```python
from build123d import *

# Parameters (mm, degrees)
F0_R     = 150
F1_DEPTH = 10
F2_R     = 150
F2_R_2   = 130
F2_R_3   = 100
F3_DEPTH = 3


with BuildPart() as f1:
    # F0 (on Top) → F1 (new body)
    with BuildSketch(Plane.XY):
        Circle(F0_R)
    extrude(amount=F1_DEPTH)

    # F2 (on face) → F3 (cut)
    with BuildSketch(Plane.XY.offset(10)):
        Circle(F2_R)
        Circle(F2_R_2, mode=Mode.SUBTRACT)
        Circle(F2_R_3)
    extrude(amount=-F3_DEPTH, mode=Mode.SUBTRACT)


solid = f1.part
```
Check sheet for the modelled part. Datum: model origin and axes. Units: mm. A direction names the side the tool comes from. Coordinates: 2 decimals unless noted, no trailing zeros. Write each loop counter-clockwise with the first axis right and the second up, starting at its lowest first coordinate (ties: lowest second). Pieces come first, ordered by that corner, then holes. Notation, with made-up numbers: (61.5, 14) -> (101.5, 14) arc R21 ccw to (101.5, 29) -> close; hole circle Ø3 at (-34, 0.25). An arc over 180 degrees is marked (long way). Use a Markdown table: item, result.
1. Sectioned sample at A-A (y = 0). Enter the section's corners in (x, z).
Reported:
| item | result |
|---|---|
| outline | (-150, 0) -> (150, 0) -> (150, 7) -> (130, 7) -> (130, 10) -> (100, 10) -> (100, 7) -> (-100, 7) -> (-100, 10) -> (-130, 10) -> (-130, 7) -> (-150, 7) -> close |
2. Tool access check on faces 4 (the flat face through (-45, 123, 7)), 5 (the cylindrical face through (-19.527, 148.724, 3.451)). Record the directions out of +Z, -Z, +X, -X, +Y, -Y that give a thin tool (end or side, any length) a straight path to the whole face; none if there is none.
Reported:
| item | result |
|---|---|
| face 4 | +Z |
| face 5 | +Z, -Z |
3. Scan lines: line 1 along Y through (x, z) = (0, 8.9); line 2 along Z through (x, y) = (-69.5, -127); line 3 along X through (y, z) = (-21.5, 7.75). Record each from-to range of solid material in increasing order.
Reported:
| item | result |
|---|---|
| line 1 | y = -130 to -100, 100 to 130 |
| line 2 | z = 0 to 7 |
| line 3 | x = -128.21 to -97.66, 97.66 to 128.21 |
4. Release check for a two-part mould opening along X. For faces 1 (the cylindrical face through (123.997, 39.048, 8.521)), 2 (the flat face through (-2, 2, 0)), 3 (the flat face through (-1, 1, 7)) record: pulls with the +X half, pulls with the -X half, needs draft (parallel to the pull), parting line crosses it, or undercut.
Reported:
| item | result |
|---|---|
| face 1 | parting line crosses it |
| face 2 | needs draft |
| face 3 | undercut |
5. Sectioned sample at C-C (z = 2.5). Enter the section's corners in (x, y).
Reported:
| item | result |
|---|---|
| outline | circle Ø300 at (0, 0) |
6. Sectioned sample at D-D (y = -120.5). Enter the section's corners in (x, z).
Reported:
| item | result |
|---|---|
| outline | (-89.33, 0) -> (89.33, 0) -> (89.33, 7) -> (48.78, 7) -> (48.78, 10) -> (-48.78, 10) -> (-48.78, 7) -> (-89.33, 7) -> close |
7. Go/stop test with flat-tipped pins: pin 1 Ø2 at (x, y) = (109.5, -35) entering from -Z; pin 2 Ø6 at (x, z) = (-84, 3) entering from -Y; pin 3 Ø5 at (y, z) = (78, 7) entering from +X; pin 4 Ø1 at (x, z) = (101, 3) entering from -Y. Record where each tip stops, or that it passes through.
Reported:
| item | result |
|---|---|
| pin 1 | stops at z = 0 |
| pin 2 | stops at y = -126.25 |
| pin 3 | stops at x = 129.61 |
| pin 4 | stops at y = -111.35 |
